```python
from build123d import *

# Parameters (mm, degrees)
BOSS_EXTRUDE2_DEPTH = 165
SKETCH2_R           = 5
CUT_EXTRUDE1_DEPTH  = 557.500817609
SKETCH3_W           = 10
SKETCH3_H           = 110
BOSS_EXTRUDE3_DEPTH = 33
BOSS_EXTRUDE4_DEPTH = 80
SKETCH5_R           = 30
CUT_EXTRUDE2_DEPTH  = 5
BOSS_EXTRUDE5_DEPTH = 7


with BuildPart() as part:
    # Sketch1 → Boss-Extrude2 (new body)
    with BuildSketch(Plane.XY):
        with BuildLine():
            Line((20, 29.6), (510, 29.6))
            ThreePointArc((510, 29.6), (517.071067812, 26.671067812), (520, 19.6))
            Line((520, 19.6), (520, 0))
            Line((520, 0), (530, 0))
            Line((530, 0), (530, 19.6))
            ThreePointArc((530, 19.6), (524.142135624, 33.742135624), (510, 39.6))
            Line((510, 39.6), (20, 39.6))
            ThreePointArc((20, 39.6), (5.857864376, 33.742135624), (0, 19.6))
            Line((0, 19.6), (0, 0))
            Line((0, 0), (10, 0))
            Line((10, 0), (10, 19.6))
            ThreePointArc((10, 19.6), (12.928932188, 26.671067812), (20, 29.6))
        make_face()
    extrude(amount=BOSS_EXTRUDE2_DEPTH)

    # Sketch2 → Cut-Extrude1 (cut, through all)
    with BuildSketch(Plane.ZY):
        with Locations((20, 10)):
            Circle(SKETCH2_R)
        with Locations(Location((145, 10, 0), (0, 0, 180))):
            Circle(SKETCH2_R)
        with Locations((75, 10)):
            Circle(SKETCH2_R)
    extrude(amount=-CUT_EXTRUDE1_DEPTH, mode=Mode.SUBTRACT)

    # Sketch3 → Boss-Extrude3 (add)
    with BuildSketch(Plane(origin=(0, 39.6, 0), x_dir=(1, 0, 0), z_dir=(0, 1, 0))):
        with Locations((225, -110)):
            Rectangle(SKETCH3_W, SKETCH3_H)
        with Locations((305, -110)):
            Rectangle(SKETCH3_W, SKETCH3_H)
    extrude(amount=BOSS_EXTRUDE3_DEPTH)

    # Sketch4 → Boss-Extrude4 (add)
    with BuildSketch(Plane(origin=(0, 0, 55), x_dir=(-1, 0, 0), z_dir=(0, 0, -1))):
        with BuildLine():
            Line((-300, 72.6), (-300, 78.6))
            ThreePointArc((-300, 78.6), (-298.828427125, 81.428427125), (-296, 82.6))
            Line((-296, 82.6), (-234, 82.6))
            ThreePointArc((-234, 82.6), (-231.171572875, 81.428427125), (-230, 78.6))
            Line((-230, 78.6), (-230, 72.6))
            Line((-230, 72.6), (-220, 72.6))
            Line((-220, 72.6), (-220, 82.6))
            ThreePointArc((-220, 82.6), (-221.464466094, 86.135533906), (-225, 87.6))
            Line((-225, 87.6), (-305, 87.6))
            ThreePointArc((-305, 87.6), (-308.535533906, 86.135533906), (-310, 82.6))
            Line((-310, 82.6), (-310, 72.6))
            Line((-310, 72.6), (-300, 72.6))
        make_face()
    extrude(amount=-BOSS_EXTRUDE4_DEPTH)

    # Sketch5 → Cut-Extrude2 (cut)
    with BuildSketch(Plane(origin=(0, 87.6, 0), x_dir=(1, 0, 0), z_dir=(0, 1, 0))):
        with Locations(Location((265, -95, 0), (0, 0, 270))):
            Circle(SKETCH5_R)
    extrude(amount=-CUT_EXTRUDE2_DEPTH, mode=Mode.SUBTRACT)

    # 3DSketch2 → Boss-Extrude5 (add)
    with BuildSketch(Plane(origin=(290, 39.6, 55), x_dir=(-0.9874406319167054, 0, 0.1579905011066729), z_dir=(0, -1, 0))):
        Polygon((0, 0), (49.372031596, 7.899525055), (50.635955605, 0), (1.263924009, -7.899525055), (0.840997387, -5.256233666), align=None)
    extrude(amount=-BOSS_EXTRUDE5_DEPTH)


solid = part.part
```
The model under review builds one solid part; all positions refer to its coordinate system, in mm. A direction names the side the tool comes from. Coordinates: 2 decimals unless noted, no trailing zeros. Write each loop counter-clockwise with the first axis right and the second up, starting at its lowest first coordinate (ties: lowest second). Pieces come first, ordered by that corner, then holes. Notation, with made-up numbers: (-5.75, 13.25) - (19.25, 13.25) arc R26 cw to (19.25, 28.25) - close; hole circle Ø2 at (12, 76.5). An arc over 180 degrees is marked (long way). Write item = value, one per line.
(1) Consider section B-B, the plane z = 145. Give the boundary of the cut face in (x, y), then the cut area to 3 significant figures.
Result sheet:
outline = (0, 0) - (10, 0) - (10, 5) - (0, 5) - close; (0, 15) - (10, 15) - (10, 19.6) arc R10 cw to (20, 29.6) - (510, 29.6) arc R10 cw to (520, 19.6) - (520, 15) - (530, 15) - (530, 19.6) arc R20 ccw to (510, 39.6) - (310, 39.6) - (310, 72.6) - (300, 72.6) - (300, 39.6) - (230, 39.6) - (230, 72.6) - (220, 72.6) - (220, 39.6) - (20, 39.6) arc R20 ccw to (0, 19.6) - close; (520, 0) - (530, 0) - (530, 5) - (520, 5) - close
area = 6,220 mm^2
(2) Consider section A-A, the plane y = 56.5. Give the boundary of the cut face in (x, z).
Result sheet:
outline = (220, 55) - (230, 55) - (230, 165) - (220, 165) - close; (300, 55) - (310, 55) - (310, 165) - (300, 165) - close
(3) Machinability: for faces 1 (the face through (4.93, 8.085, 79.619)), 2 (the face through (305, 72.6, 150)), 3 (the face through (12.85, 26.59, 81.34)), which of the approach directions +Z, -Z, +X, -X, +Y, -Y give a long, thin tool a straight path to every point of the face, cutting with its end or side? Answer none if there is none.
Result sheet:
face_1 = +X, -X
face_2 = +Z, +X, -X, +Y
face_3 = +Z, -Z, -Y
(4) Mouldability with a two-part tool opening along Z and no side actions: class faces 4 (the face through (266, 84, 135)), 5 (the face through (4.93, 14.957, 19.349)), 6 (the face through (524.93, 8.085, 79.619)), 7 (the face through (251.7, 82.6, 67.8)) as pulls with the +Z half, pulls with the -Z half, needs draft (parallel to the pull), parting line crosses it, or undercut.
Result sheet:
face_4 = pulls with the +Z half
face_5 = undercut
face_6 = undercut
face_7 = needs draft
(5) Consider section D-D, the plane y = 10. State how many separate pieces and enclosed holes the cut face has, then the cut area to 3 significant figures.
Result sheet:
separate_pieces = 8
enclosed_holes = 0
area = 2,700 mm^2
(6) For line 1 (X direction, y = 78, z = 100.5); line 2 (Y direction, x = 453.5, z = 89); line 3 (Y direction, x = 4.5, z = 145), list the stretches that pass through material, from the lowest coordinate up. Write a range as [from, to].
Result sheet:
line_1 = [220, 230], [300, 310]
line_2 = [29.6, 39.6]
line_3 = [0, 5], [15, 32.24]
(7) For P1, Ø6, axis at y = 44.5, z = 59, coming from the +X side; P2, Ø11, axis at x = 303, z = 152, coming from the +Y side; P3, Ø24, axis at x = 283.5, y = 63, coming from the -Z side; P4, Ø16.5, axis at x = 248.5, y = 82.5, coming from the +Z side, all flat-tipped, find the tip position at first contact; note any pin that passes through.
Result sheet:
P1 = 310
P2 = 72.6
P3 = through
P4 = 135
(8) Consider section C-C, the plane x = 265. Give the boundary of the cut face in (y, z).
Result sheet:
outline = (29.6, 0) - (39.6, 0) - (39.6, 55) - (46.6, 55) - (46.6, 63) - (39.6, 63) - (39.6, 165) - (29.6, 165) - close; (82.6, 55) - (87.6, 55) - (87.6, 65) - (82.6, 65) - close; (82.6, 125) - (87.6, 125) - (87.6, 135) - (82.6, 135) - close
